Work out the finished part from the listing and answer in its coordinate system (mm). A direction names the side the tool comes from. Coordinates: 2 decimals unless noted, no trailing zeros. Loops run counter-clockwise (first coordinate to the right, second up) from the corner with the lowest first, then second, coordinate; pieces in that order, holes last. Notation, with made-up numbers: (1, 77) - (55, 77) arc R19 cw to (55, 102) - close; hole circle Ø9 at (-25, 12.25). An arc over 180 degrees is marked (long way). Write each question's results on one line, items separated by ' | '. Start each with the question number.
1. A cutting plane is placed at B-B on z = 21.5. Determine the outline of the cut face in (x, y), then the cut area to 3 significant figures.
2. Find the intervals of material crossed by line 1 along X through (y, z) = (-83.5, 19.5); line 2 along Y through (x, z) = (75, 30); line 3 along Y through (x, z) = (75, 6.5), in increasing order. Write a range as [from, to].
3. A cutting plane is placed at C-C on x = -16. Determine the outline of the cut face in (y, z), then the cut area to 3 significant figures.
4. Which of the six approach directions +Z, -Z, +X, -X, +Y, -Y give full straight-line access (tool end or side, diameter ignored) to faces 1 (the flat face through (-47, 14.5, 104)), 2 (the flat face through (68, -86, 24.9)), 3 (the flat face through (-1, -112.5, 23)), 4 (the flat face through (68, -69, 35)), 5 (the flat face through (23, -31, 5))?
5. Determine the mould class of faces 6 (the cylindrical face through (93.15, 36.49, 14.86)), 7 (the flat face through (72, 48.5, 52)), 8 (the cylindrical face through (-101.99, 109.65, 12.68)) for opening direction X: released by +X, released by -X, zero draft, split by the parting line, or undercut.
6. A cutting plane is placed at D-D on x = -89.5. Determine the outline of the cut face in (y, z).
7. Each of these flat-tipped pins is pushed along its axis until it touches: P1, Ø8, axis at y = -91, z = 38.5, coming from the +X side; P2, Ø12, axis at x = -54, y = 5.5, coming from the -Z side; P3, Ø1.5, axis at y = -46.5, z = 137, coming from the -X side; P4, Ø2, axis at y = -87.5, z = 110.5, coming from the -X side. Where does it stop, or does it pass through?
8. A cutting plane is placed at A-A on y = -82.5. Determine the outline of the cut face in (x, z), then the cut area to 3 significant figures.
from build123d import *

# Parameters (mm, degrees)
F0_W            = 210
F0_H            = 225
F1_DEPTH        = 25
F3_DEPTH        = 95
F4_R            = 37.5
F5_DEPTH        = 10
F5_DEPTH_BACK   = 127
F6_R            = 40
F7_DEPTH        = 10
F7_DEPTH_BACK   = 127
F8_W            = 60
F8_H            = 60
F9_DEPTH        = 10
F10_R           = 10
F12_DEPTH       = 20
F14_D           = 15
F14_CBORE_D     = 30
F14_CBORE_DEPTH = 10.1
F15_R           = 10
F16_R           = 10
F17_R           = 19.5
F18_DEPTH       = 235.001
F19_R           = 19.5
F20_DEPTH       = 220.001
F21_SIZE        = 2
F22_R           = 10


with BuildPart() as f1:
    # F0 (on Top) → F1 (new body)
    with BuildSketch(Plane.XY):
        Rectangle(F0_W, F0_H)
    extrude(amount=F1_DEPTH)

    # F2 (on face) → F3 (join)
    with BuildSketch(Plane.XY.offset(25)):
        with BuildLine():
            Line((-71, -32.5), (-71, -112.5))
            Line((-71, -112.5), (-56.000001, -112.5))
            Line((-56.000001, -112.5), (-56.000001, -46.481815))
            ThreePointArc((-56.000001, -46.481815), (7.488852, -14.988852), (38.981815, 48.500001))
            Line((38.981815, 48.500001), (105, 48.500001))
            Line((105, 48.500001), (105, 63.5))
            Line((105, 63.5), (25, 63.5))
            ThreePointArc((25, 63.5), (-3.117749, -4.382251), (-71, -32.5))
        make_face()
    extrude(amount=F3_DEPTH)

    # F4 (on face) → F5 (join, two sides)
    with BuildSketch(Plane.XZ.offset(112.5)) as f5_sk:
        with Locations((-63.500001, 120)):
            Circle(F4_R)
    extrude(amount=F5_DEPTH)
    extrude(f5_sk.sketch, amount=-F5_DEPTH_BACK)

    # F6 (on face) → F7 (join, two sides)
    with BuildSketch(Plane.YZ.offset(105)) as f7_sk:
        with Locations((56.000001, 120)):
            Circle(F6_R)
    extrude(amount=F7_DEPTH)
    extrude(f7_sk.sketch, amount=-F7_DEPTH_BACK)

    # F8 (on face) → F9 (join)
    with BuildSketch(Plane.XY.offset(25)):
        with Locations((75, -82.5)):
            Rectangle(F8_W, F8_H)
    extrude(amount=F9_DEPTH)

    # F10
    f10_edges = [f1.edges().sort_by_distance(p)[0] for p in [
        (45, -52.5, 30),
    ]]
    fillet(f10_edges, radius=F10_R)

    # F11 (on face) → F12 (cut)
    with BuildSketch(Plane.XY.offset(25)):
        with BuildLine():
            ThreePointArc((46.575506, 39.500003), (13.852812, -21.352812), (-47.000003, -54.075506))
            Line((-47.000003, -54.075506), (-47.000003, -103.500001))
            Line((-47.000003, -103.500001), (36.000001, -103.500001))
            Line((36.000001, -103.500001), (36.000001, -62.5))
            ThreePointArc((36.000001, -62.5), (41.564972, -49.064972), (55, -43.500001))
            Line((55, -43.500001), (96.000001, -43.500001))
            Line((96.000001, -43.500001), (96.000001, 39.500003))
            Line((96.000001, 39.500003), (46.575506, 39.500003))
        make_face()
    extrude(amount=-F12_DEPTH, mode=Mode.SUBTRACT)

    # F14 (through all)
    with Locations(Plane.XY.offset(35)):
        with Locations((75, -82.5)):
            CounterBoreHole(F14_D / 2, F14_CBORE_D / 2, F14_CBORE_DEPTH)

    # F15
    f15_edges = [f1.edges().sort_by_distance(p)[0] for p in [
        (-47.000003, -54.075506, 15),
        (46.575506, 39.500003, 15),
        (-47.000003, -103.500001, 15),
        (96.000001, 39.500003, 15),
    ]]
    fillet(f15_edges, radius=F15_R)

    # F16
    f16_edges = [f1.edges().sort_by_distance(p)[0] for p in [
        (96.000001, -43.500001, 15),
        (36.000001, -103.500001, 15),
    ]]
    fillet(f16_edges, radius=F16_R)

    # F17 (on face) → F18 (cut, through all)
    with BuildSketch(Plane.XZ.offset(122.5)):
        with Locations((-63.500001, 120)):
            Circle(F17_R)
    extrude(amount=-F18_DEPTH, mode=Mode.SUBTRACT)

    # F19 (on face) → F20 (cut, through all)
    with BuildSketch(Plane.YZ.offset(115)):
        with Locations((56.000001, 120)):
            Circle(F19_R)
    extrude(amount=-F20_DEPTH, mode=Mode.SUBTRACT)

    # F21
    f21_edges = [f1.edges().sort_by_distance(p)[0] for p in [
        (115, 36.500001, 120),
        (-83.000001, -122.5, 120),
        (-22, 36.500001, 120),
        (-83.000001, 14.5, 120),
    ]]
    chamfer(f21_edges, length=F21_SIZE)

    # F22
    f22_edges = [f1.edges().sort_by_distance(p)[0] for p in [
        (-105, -112.5, 12.5),
        (105, -112.5, 17.5),
        (105, 112.5, 12.5),
        (-105, 112.5, 12.5),
    ]]
    fillet(f22_edges, radius=F22_R)


solid = f1.part
Values:
1) outline: (-105, -102.5) arc R10 ccw to (-95, -112.5) - (95, -112.5) arc R10 ccw to (105, -102.5) - (105, 102.5) arc R10 ccw to (95, 112.5) - (-95, 112.5) arc R10 ccw to (-105, 102.5) - close; hole (-47, -93.5) arc R10 ccw to (-37, -103.5) - (26, -103.5) arc R10 ccw to (36, -93.5) - (36, -62.5) arc R19 cw to (55, -43.5) - (86, -43.5) arc R10 ccw to (96, -33.5) - (96, 29.5) arc R10 ccw to (86, 39.5) - (54.48, 39.5) arc R10 ccw to (44.82, 32.12) arc R120 cw to (-39.62, -52.32) arc R10 ccw to (-47, -61.98) - close; hole circle Ø15 at (75, -82.5) | area: 36,300 mm^2
2) line 1: [-105, -47], [36, 67.57], [82.43, 105] | line 2: [-112.5, -97.5], [-67.5, -52.5], [48.5, 63.5] | line 3: [-112.5, -90], [-75, -43.5], [39.5, 112.5]
3) outline: (-112.5, 0) - (112.5, 0) - (112.5, 25) - (-15.18, 25) - (-15.18, 120) - (-32.92, 120) - (-32.92, 25) - (-43.15, 25) - (-43.15, 5) - (-103.5, 5) - (-103.5, 25) - (-112.5, 25) - close; circle Ø80 at (56, 120); hole circle Ø39 at (56, 120) | area: 9,930 mm^2
4) face 1: +Z, -X, +Y | face 2: +Z | face 3: -Z, +X, -X, -Y | face 4: +Z, +X, -Y | face 5: none
5) face 6: undercut | face 7: zero draft | face 8: released by -X
6) outline: (-122.5, 92.98) - (14.5, 92.98) - (14.5, 147.02) - (-122.5, 147.02) - close; (-112.5, 0) - (112.5, 0) - (112.5, 25) - (-112.5, 25) - close
7) P1: x = 105 | P2: z = 0 | P3: x = -97.3 | P4: x = -100.02
8) outline: (-105, 0) - (67.5, 0) - (67.5, 24.9) - (60, 24.9) - (60, 35) - (45, 35) - (45, 25) - (36, 25) - (36, 5) - (-47, 5) - (-47, 25) - (-56, 25) - (-56, 83.26) arc R37.5 ccw (long way) to (-71, 83.26) - (-71, 25) - (-105, 25) - close; (82.5, 0) - (105, 0) - (105, 35) - (90, 35) - (90, 24.9) - (82.5, 24.9) - close; hole circle Ø39 at (-63.5, 120) | area: 7,600 mm^2
